from build123d import *

# Parameters (mm, degrees)
F0_R     = 5.969
F1_DEPTH = 6.35
F3_DEPTH = 3.175
F4_R     = 5.969
F5_DEPTH = 3.175
F6_R     = 2.38125
F7_DEPTH = 25.4


with BuildPart() as f1:
    # F0 (on Front) → F1 (new body)
    with BuildSketch(Plane.XZ):
        with BuildLine():
            ThreePointArc((-3.193241, 25.198476), (21.997045, 12.7), (20.2259, -15.364666))
            Line((20.2259, -15.364666), (30.925328, -33.896619))
            ThreePointArc((30.925328, -33.896619), (34.982408, -33.229802), (39.025166, -32.481036))
            ThreePointArc((39.025166, -32.481036), (46.72867, -26.97881), (47.641985, -17.556267))
            ThreePointArc((47.641985, -17.556267), (31.40528, 18.131847), (8.616819, 50.037303))
            ThreePointArc((8.616819, 50.037303), (0, 53.957621), (-8.616819, 50.037303))
            ThreePointArc((-8.616819, 50.037303), (-11.286649, 46.910555), (-13.892669, 43.73043))
            Line((-13.892669, 43.73043), (-3.193241, 25.198476))
        make_face()
        with Locations((36.83, -21.26381)):
            Circle(F0_R, mode=Mode.SUBTRACT)
        with Locations((0, 42.527621)):
            Circle(F0_R, mode=Mode.SUBTRACT)
    extrude(amount=F1_DEPTH)

    # F2 (on face) → F3 (cut)
    with BuildSketch(Plane.XZ.offset(6.35)):
        Polygon((-39.208766, 26.267834), (-6.944216, 7.639887), (20.571818, 55.299056), (-11.692732, 73.927002), align=None)
    extrude(amount=-F3_DEPTH, mode=Mode.SUBTRACT)

    # F4 (on face) → F5 (cut)
    with BuildSketch(Plane.XZ):
        with Locations((36.83, -21.26381)):
            Circle(F4_R)
        with BuildLine():
            Line((65.582015, -59.232034), (65.582015, -9.83381))
            Line((65.582015, -9.83381), (44.817998, -9.83381))
            ThreePointArc((44.817998, -9.83381), (46.269057, -13.680753), (47.641985, -17.556267))
            ThreePointArc((47.641985, -17.556267), (46.72867, -26.97881), (39.025166, -32.481036))
            ThreePointArc((39.025166, -32.481036), (34.982408, -33.229802), (30.925328, -33.896619))
            Line((30.925328, -33.896619), (20.2259, -15.364666))
            ThreePointArc((20.2259, -15.364666), (21.997045, -12.7), (23.419141, -9.83381))
            Line((23.419141, -9.83381), (1.765535, -9.83381))
            Line((1.765535, -9.83381), (1.765535, -59.232034))
            Line((1.765535, -59.232034), (65.582015, -59.232034))
        make_face()
        with BuildLine():
            ThreePointArc((47.641985, -17.556267), (46.269057, -13.680753), (44.817998, -9.83381))
            Line((44.817998, -9.83381), (23.419141, -9.83381))
            ThreePointArc((23.419141, -9.83381), (21.997045, -12.7), (20.2259, -15.364666))
            Line((20.2259, -15.364666), (30.925328, -33.896619))
            ThreePointArc((30.925328, -33.896619), (34.982408, -33.229802), (39.025166, -32.481036))
            ThreePointArc((39.025166, -32.481036), (46.72867, -26.97881), (47.641985, -17.556267))
        make_face()
        with Locations((36.83, -21.26381)):
            Circle(F4_R, mode=Mode.SUBTRACT)
    extrude(amount=F5_DEPTH, mode=Mode.SUBTRACT)

    # F6 (on face) → F7 (cut)
    with BuildSketch(Plane.XZ.offset(6.35)):
        with Locations((28.349303, 12.88107)):
            Circle(F6_R)
    extrude(amount=-F7_DEPTH, mode=Mode.SUBTRACT)


solid = f1.part
The model under review builds one solid part; all positions refer to its coordinate system, in mm. A direction names the side the tool comes from. Round coordinates to 2 decimals unless told otherwise and drop trailing zeros. Order: outer loops, then holes, each group sorted by start corner. A loop starts at its lowest first (then second) coordinate and runs counter-clockwise, first axis right, second up. Notation, with made-up numbers: (55.5, 2) - (109.5, 2) arc R31 cw to (109.5, 29) - close; hole circle Ø1 at (77.5, 78.25). An arc over 180 degrees is marked (long way). Use one line per item in the form item = value.
Q1. Add section C-C on y = -1.5. Give the boundary of the cut face in (x, z), then the cut area to 3 significant figures.
Response values:
outline = (-13.89, 43.73) - (-3.19, 25.2) arc R25.4 cw to (23.42, -9.83) - (44.82, -9.83) arc R203.2 ccw to (8.62, 50.04) arc R11.43 ccw to (-8.62, 50.04) arc R203.2 ccw to start; hole circle Ø11.94 at (0, 42.53); hole circle Ø4.76 at (28.35, 12.88)
area = 1,140 mm^2
Q2. Add section B-B on x = 0. Give the boundary of the cut face in (y, z) (3 decimals).
Response values:
outline = (-3.175, 25.4) - (0, 25.4) - (0, 36.559) - (-3.175, 36.559) - close; (-3.175, 48.497) - (0, 48.497) - (0, 53.958) - (-3.175, 53.958) - close
Q3. Tool access review of faces 5 (the flat face through (3, -3.175, 37)), 6 (the flat face through (31, -3.175, -19)), 7 (the cylindrical face through (46.66, -4.74, -27.1)): name each direction out of +Z, -Z, +X, -X, +Y, -Y from which nothing blocks a thin tool from reaching the whole face with its end or side.
Response values:
face_5 = +Z, -X, -Y
face_6 = -Z, +X, -X, +Y
face_7 = +X, +Y, -Y
Q4. To check wall thickness, follow line 1 (Z direction, x = 0, y = -1.9); line 2 (Z direction, x = 0.5, y = -1.25); line 3 (Y direction, x = -9, z = 43) (3 decimals). State the ranges of each line that lie inside material, in increasing order.
Response values:
line_1 = 25.4 to 36.56, 48.5 to 53.96
line_2 = 25.4 to 36.58, 48.48 to 53.95
line_3 = -3.175 to 0
Q5. Add section D-D on z = -22.5. Give the boundary of the cut face in (x, y) (3 decimals), then the cut area to 3 significant figures.
Response values:
outline = (24.345, -6.35) - (30.99, -6.35) - (30.99, -3.175) - (24.345, -3.175) - close; (42.67, -6.35) - (48.193, -6.35) - (48.193, -3.175) - (42.67, -3.175) - close
area = 38.6 mm^2
Q6. Add section A-A on z = 40.5. Give the boundary of the cut face in (x, y) (3 decimals).
Response values:
outline = (-12.028, -3.175) - (-5.614, -3.175) - (-5.614, 0) - (-12.028, 0) - close; (5.614, -3.175) - (12.028, -3.175) - (12.028, -6.35) - (16.432, -6.35) - (16.432, 0) - (5.614, 0) - close
Q7. Clearance check with flat-ended pins moving along their axes: P1, Ø1, axis at x = 23, z = 28, coming from the +Y side; P2, Ø13.5, axis at x = 36.83, z = -21.26, coming from the +Y side (3 decimals); P3, Ø1.6, axis at x = 36.5, y = -1.5, coming from the -Z side. State where each tip first meets the part, or that it passes through.
Response values:
P1 = 0
P2 = -3.175
P3 = -9.83
Q8. Mouldability with a two-part tool opening along X and no side actions: class faces 1 (the cylindrical face through (31.68, -3.131, 17.655)), 2 (the cylindrical face through (2.75, -1.57, 37.23)), 3 (the flat face through (25.5, -4.7, -24.5)), 4 (the cylindrical face through (39.58, -4.74, -26.56)) as pulls with the +X half, pulls with the -X half, needs draft (parallel to the pull), parting line crosses it, or undercut.
Response values:
face_1 = pulls with the +X half
face_2 = undercut
face_3 = pulls with the -X half
face_4 = undercut
